Verification items for the finished model (mm, model axes). Round coordinates to 2 decimals unless told otherwise and drop trailing zeros. Write each loop counter-clockwise with the first axis right and the second up, starting at its lowest first coordinate (ties: lowest second). Pieces come first, ordered by that corner, then holes.
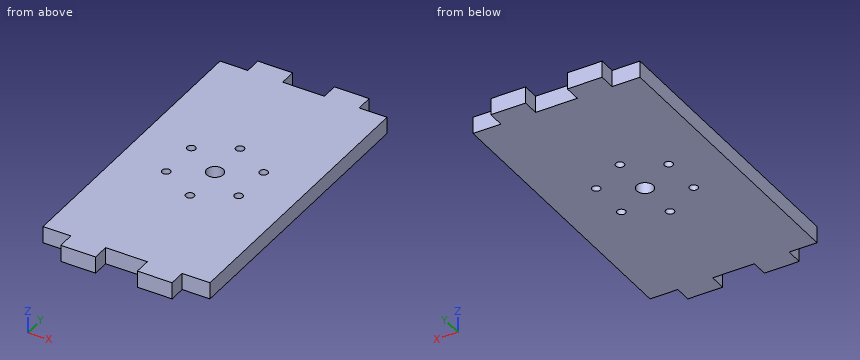
from build123d import *

# Parameters (mm, degrees)
SKETCH1_R           = 0.75
SKETCH1_R_2         = 1.5
BOSS_EXTRUDE1_DEPTH = 3


with BuildPart() as part:
    # Sketch1 → Boss-Extrude1 (new body)
    with BuildSketch(Plane.XY):
        Polygon((-15, 26.5), (-10, 26.5), (-10, 29.5), (-3.75, 29.5), (-3.75, 26.5), (3.75, 26.5), (3.75, 29.5), (10, 29.5), (10, 26.5), (15, 26.5), (15, -26.5), (10, -26.5), (10, -29.5), (3.75, -29.5), (3.75, -26.5), (-3.75, -26.5), (-3.75, -29.5), (-10, -29.5), (-10, -26.5), (-15, -26.5), align=None)
        with Locations((0, 7.5)):
            Circle(SKETCH1_R, mode=Mode.SUBTRACT)
        with Locations((6.495190528, 3.75)):
            Circle(SKETCH1_R, mode=Mode.SUBTRACT)
        with Locations((6.495190528, -3.75)):
            Circle(SKETCH1_R, mode=Mode.SUBTRACT)
        with Locations((0, -7.5)):
            Circle(SKETCH1_R, mode=Mode.SUBTRACT)
        with Locations((-6.495190528, -3.75)):
            Circle(SKETCH1_R, mode=Mode.SUBTRACT)
        with Locations((-6.495190528, 3.75)):
            Circle(SKETCH1_R, mode=Mode.SUBTRACT)
        Circle(SKETCH1_R_2, mode=Mode.SUBTRACT)
    extrude(amount=BOSS_EXTRUDE1_DEPTH)


solid = part.part
Q1. Sectioned sample at A-A (y = 3.75). Enter the section's corners in (x, z), plus the area to 3 significant figures.
Recorded:
outline: (-15, 0) - (-7.25, 0) - (-7.25, 3) - (-15, 3) - close; (-5.75, 0) - (5.75, 0) - (5.75, 3) - (-5.75, 3) - close; (7.25, 0) - (15, 0) - (15, 3) - (7.25, 3) - close
area: 81.0 mm2
Q2. Depth check by flat-ended pin: P1, Ø1.5, axis at y = 28.5, z = 2, coming from the -X side; P2, Ø1.7, axis at x = 6.5, y = 3.75, coming from the -Z side; P3, Ø0.9, axis at y = 27.5, z = 1, coming from the +X side; P4, Ø1.5, axis at x = 13, z = 1.5, coming from the +Y side. Enter the tip coordinate at first touch or a pass-through.
Recorded:
P1: stops at x = -10
P2: stops at z = 0
P3: stops at x = 10
P4: stops at y = 26.5
Q3. Sectioned sample at D-D (z = 1.8). Enter the section's corners in (x, y), plus the area to 3 significant figures.
Recorded:
outline: (-15, -26.5) - (-10, -26.5) - (-10, -29.5) - (-3.75, -29.5) - (-3.75, -26.5) - (3.75, -26.5) - (3.75, -29.5) - (10, -29.5) - (10, -26.5) - (15, -26.5) - (15, 26.5) - (10, 26.5) - (10, 29.5) - (3.75, 29.5) - (3.75, 26.5) - (-3.75, 26.5) - (-3.75, 29.5) - (-10, 29.5) - (-10, 26.5) - (-15, 26.5) - close; hole circle Ø1.5 at (-6.5, -3.75); hole circle Ø1.5 at (-6.5, 3.75); hole circle Ø3 at (0, 0); hole circle Ø1.5 at (0, -7.5); hole circle Ø1.5 at (0, 7.5); hole circle Ø1.5 at (6.5, -3.75); hole circle Ø1.5 at (6.5, 3.75)
area: 1,650 mm2
Q4. Material ranges on line 1 along Y through (x, z) = (0, 1.3); line 2 along Y through (x, z) = (0.5, 1.1); line 3 along Y through (x, z) = (-11.75, 0.5), recorded low to high.
Recorded:
line 1: y = -26.5 to -8.25, -6.75 to -1.5, 1.5 to 6.75, 8.25 to 26.5
line 2: y = -26.5 to -8.06, -6.94 to -1.41, 1.41 to 6.94, 8.06 to 26.5
line 3: y = -26.5 to 26.5
Q5. Sectioned sample at B-B (x = 0). Enter the section's corners in (y, z), plus the area to 3 significant figures.
Recorded:
outline: (-26.5, 0) - (-8.25, 0) - (-8.25, 3) - (-26.5, 3) - close; (-6.75, 0) - (-1.5, 0) - (-1.5, 3) - (-6.75, 3) - close; (1.5, 0) - (6.75, 0) - (6.75, 3) - (1.5, 3) - close; (8.25, 0) - (26.5, 0) - (26.5, 3) - (8.25, 3) - close
area: 141 mm2
Q6. Sectioned sample at C-C (y = -7.5). Enter the section's corners in (x, z), plus the area to 3 significant figures.
Recorded:
outline: (-15, 0) - (-0.75, 0) - (-0.75, 3) - (-15, 3) - close; (0.75, 0) - (15, 0) - (15, 3) - (0.75, 3) - close
area: 85.5 mm2
